Check sheet for the modelled part. Datum: model origin and axes. Units: mm. A direction names the side the tool comes from. Give positions to 0.01 mm unless a question says otherwise; leave off trailing zeros. Write each loop counter-clockwise with the first axis right and the second up, starting at its lowest first coordinate (ties: lowest second). Pieces come first, ordered by that corner, then holes. Notation, with made-up numbers: (-21.75, 29) -> (9.25, 29) arc R23 ccw to (9.25, 54) -> close; hole circle Ø3 at (34, 50). An arc over 180 degrees is marked (long way). Return JSON: item names as keys, results as strings.
from build123d import *

# Parameters (mm, degrees)
BOSS_EXTRUDE1_DEPTH            = 12
SKETCH41_R                     = 1.71
CUT_EXTRUDE7_DEPTH             = 18
CBORE_FOR_M3_SHCS1_D           = 3.4
CBORE_FOR_M3_SHCS1_CBORE_D     = 6.5
CBORE_FOR_M3_SHCS1_CBORE_DEPTH = 3
CBORE_FOR_M3_SHCS2_D           = 3.4
CBORE_FOR_M3_SHCS2_CBORE_D     = 6.5
CBORE_FOR_M3_SHCS2_CBORE_DEPTH = 3
CUT_EXTRUDE10_DEPTH            = 15
CUT_EXTRUDE10_DEPTH_BACK       = 15
SKETCH52_R                     = 1.7
SKETCH58_R                     = 3.25
CUT_EXTRUDE11_DEPTH            = 8
CUT_EXTRUDE12_DEPTH            = 4
CUT_EXTRUDE12_DEPTH_BACK       = 6
FILLET1_R                      = 2
SKETCH61_R                     = 3.25
CUT_EXTRUDE13_DEPTH            = 6
CUT_EXTRUDE14_DEPTH            = 1


with BuildPart() as part:
    # Sketch1 → Boss-Extrude1 (new body)
    with BuildSketch(Plane(origin=(0, 0, 0), x_dir=(0, 1, 0), z_dir=(0, 0, 1))):
        with BuildLine():
            Line((-6.350852961, -13), (13.279056191, -13))
            Line((13.279056191, -13), (13.279056191, -1))
            Line((13.279056191, -1), (3.97617907, -1))
            ThreePointArc((3.97617907, -1), (3.601659304, -1.959094244), (3, -2.794637722))
            Line((3, -2.794637722), (-3, -2.794637722))
            ThreePointArc((-3, -2.794637722), (-3.815101571, -1.501665742), (-4.1, 0))
            ThreePointArc((-4.1, 0), (-0.503818326, 4.06892702), (3.97617907, 1))
            Line((3.97617907, 1), (13.279056191, 1))
            Line((13.279056191, 1), (13.279056191, 13))
            Line((13.279056191, 13), (-6.350852961, 13))
            Line((-6.350852961, 13), (-13.856406461, 0))
            Line((-13.856406461, 0), (-6.350852961, -13))
        make_face()
    extrude(amount=BOSS_EXTRUDE1_DEPTH)

    # Sketch41 → Cut-Extrude7 (cut)
    with BuildSketch(Plane(origin=(0, 0, 0), x_dir=(0, 1, 0), z_dir=(0, 0, 1))):
        with Locations(Location((0, 8.6, 0), (0, 0, 270))):
            Circle(SKETCH41_R)
        with Locations(Location((0, -8.6, 0), (0, 0, 270))):
            Circle(SKETCH41_R)
    extrude(amount=CUT_EXTRUDE7_DEPTH, mode=Mode.SUBTRACT)

    # CBORE for M3 SHCS1 (through all)
    with Locations(Plane(origin=(-8.6, 0, 12), x_dir=(1, 0, 0), z_dir=(0, 0, 1))):
        with Locations((0, 0)):
            CounterBoreHole(CBORE_FOR_M3_SHCS1_D / 2, CBORE_FOR_M3_SHCS1_CBORE_D / 2, CBORE_FOR_M3_SHCS1_CBORE_DEPTH)

    # CBORE for M3 SHCS2 (through all)
    with Locations(Plane(origin=(8.6, 0, 12), x_dir=(1, 0, 0), z_dir=(0, 0, 1))):
        with Locations((0, 0)):
            CounterBoreHole(CBORE_FOR_M3_SHCS2_D / 2, CBORE_FOR_M3_SHCS2_CBORE_D / 2, CBORE_FOR_M3_SHCS2_CBORE_DEPTH)

    # Sketch52 → Cut-Extrude10 (cut, two sides: drawn at the far end of the back side and taken through both)
    with BuildSketch(Plane.YZ.offset(-1).offset(-CUT_EXTRUDE10_DEPTH_BACK)):
        with Locations((8.106406461, 6)):
            Circle(SKETCH52_R)
    extrude(amount=CUT_EXTRUDE10_DEPTH + CUT_EXTRUDE10_DEPTH_BACK, mode=Mode.SUBTRACT)

    # Sketch58 → Cut-Extrude11 (cut)
    with BuildSketch(Plane.YZ.offset(13)):
        with Locations(Location((8.106406461, 6, 0), (0, 0, 270))):
            Circle(SKETCH58_R)
    extrude(amount=-CUT_EXTRUDE11_DEPTH, mode=Mode.SUBTRACT)

    # Sketch60 → Cut-Extrude12 (cut, two sides: drawn at the far end of the back side and taken through both)
    with BuildSketch(Plane.YZ.offset(-8).offset(-CUT_EXTRUDE12_DEPTH_BACK)):
        Polygon((8.106406461, 2.709103466), (10.956406461, 4.354551733), (10.956406461, 7.645448267), (8.106406461, 9.290896534), (5.256406461, 7.645448267), (5.256406461, 4.354551733), align=None)
    extrude(amount=CUT_EXTRUDE12_DEPTH + CUT_EXTRUDE12_DEPTH_BACK, mode=Mode.SUBTRACT)

    # Fillet1
    # the kernel refuses this fillet: 2 mm, written as the material it takes off along each edge
    with BuildSketch(Plane(origin=(13, 13.279056191, -5), x_dir=(0, -1, 0), z_dir=(0, 0, 1))) as fillet1_piece_1:
        with BuildLine():
            CenterArc((FILLET1_R, -FILLET1_R), FILLET1_R, 90, 90)
            Line((0, -FILLET1_R), (0, 0))
            Line((0, 0), (FILLET1_R, 0))
        make_face()
    extrude(amount=22, mode=Mode.SUBTRACT)
    with BuildSketch(Plane(origin=(-13, 13.279056191, -5), x_dir=(0, -1, 0), z_dir=(0, 0, 1))) as fillet1_piece_2:
        with BuildLine():
            CenterArc((FILLET1_R, FILLET1_R), FILLET1_R, 180, 90)
            Line((0, FILLET1_R), (0, 0))
            Line((0, 0), (FILLET1_R, 0))
        make_face()
    extrude(amount=22, mode=Mode.SUBTRACT)

    # Sketch61 → Cut-Extrude13 (cut)
    with BuildSketch(Plane(origin=(0, 0, 12), x_dir=(0, 1, 0), z_dir=(0, 0, 1))):
        with Locations(Location((0, 8.6, 0), (0, 0, 270))):
            Circle(SKETCH61_R)
        with Locations(Location((0, -8.6, 0), (0, 0, 270))):
            Circle(SKETCH61_R)
    extrude(amount=-CUT_EXTRUDE13_DEPTH, mode=Mode.SUBTRACT)

    # Sketch62 → Cut-Extrude14 (cut)
    with BuildSketch(Plane(origin=(-6, -10.392304845, 0), x_dir=(0.8660254037844386, -0.5000000000000001, 0), z_dir=(-0.5000000000000001, -0.8660254037844386, 0))):
        with BuildLine():
            Line((1.681473513, 6.646959362), (1.681473513, 6.287985003))
            Line((1.681473513, 6.287985003), (0.491669827, 6.287985003))
            Line((0.491669827, 6.287985003), (0.302366943, 5.367412086))
            add(Edge.make_bspline(
                [(0.302366943, 5.367412086), (0.339422817, 5.377642358), (0.411212713, 5.397461892), (0.517172574, 5.419467662), (0.617764777, 5.432733106), (0.683040148, 5.434544417), (0.714626558, 5.435420901)],
                knots=[0, 0, 0, 0, 1.100273476, 2.13160584, 3.095893838, 4, 4, 4, 4], degree=3))
            add(Edge.make_bspline(
                [(0.714626558, 5.435420901), (0.753710298, 5.434574965), (0.830558695, 5.432911644), (0.942997642, 5.416939795), (1.050330535, 5.39179988), (1.152332906, 5.356679358), (1.249193456, 5.311769625), (1.340021018, 5.255669685), (1.426178931, 5.190136353), (1.506121525, 5.114791341), (1.578645833, 5.031869725), (1.642411822, 4.942711854), (1.696574413, 4.848184192), (1.740135168, 4.747383583), (1.774919502, 4.641424429), (1.798071497, 4.529191847), (1.813488206, 4.411743727), (1.815210592, 4.331439157), (1.816088898, 4.29048901)],
                knots=[0, 0, 0, 0, 1.052922333, 2.070308379, 3.05430497, 4.020497103, 4.973039431, 5.925935799, 6.892292201, 7.88610001, 8.88166317, 9.857072816, 10.836096531, 11.812156883, 12.81219415, 13.836441305, 14.89672472, 16, 16, 16, 16], degree=3))
            add(Edge.make_bspline(
                [(1.816088898, 4.29048901), (1.815423823, 4.261966789), (1.81410266, 4.205307802), (1.807384072, 4.121163601), (1.794448356, 4.038800768), (1.777080632, 3.958208376), (1.754538214, 3.879539004), (1.72724916, 3.802567476), (1.693853133, 3.727772869), (1.657221758, 3.654447474), (1.61597528, 3.584248967), (1.570196772, 3.51859998), (1.521831281, 3.456515699), (1.469789896, 3.398661966), (1.4135889, 3.345418948), (1.353908934, 3.296470667), (1.291226215, 3.250989336), (1.224570972, 3.210821141), (1.155428489, 3.173858185), (1.082800272, 3.143534648), (1.008339572, 3.116424119), (0.930974696, 3.094814592), (0.850880883, 3.077882037), (0.767926108, 3.066381437), (0.682545438, 3.058004999), (0.624670425, 3.057480642), (0.595435853, 3.057215772)],
                knots=[0, 0, 0, 0, 1.056347294, 2.098418968, 3.122841568, 4.141288669, 5.149314143, 6.15115421, 7.162517403, 8.180376062, 9.185164535, 10.17417709, 11.141909838, 12.097768115, 13.052685741, 14.0056014, 14.954263652, 15.917497458, 16.885230207, 17.854509472, 18.828990115, 19.81800267, 20.826176721, 21.857883937, 22.917946725, 24, 24, 24, 24], degree=3))
            add(Edge.make_bspline(
                [(0.595435853, 3.057215772), (0.560561672, 3.05790661), (0.491950842, 3.059265752), (0.391430275, 3.073484238), (0.294715669, 3.093848154), (0.202585568, 3.124484424), (0.114214304, 3.162871719), (0.030791586, 3.21138789), (-0.04981419, 3.266366994), (-0.124326227, 3.331247347), (-0.19348234, 3.402163029), (-0.255388849, 3.47912067), (-0.310522426, 3.560850112), (-0.358000173, 3.647748266), (-0.398498194, 3.739586797), (-0.430313182, 3.836709798), (-0.455991537, 3.938609802), (-0.466854958, 4.008763312), (-0.472372641, 4.04439526)],
                knots=[0, 0, 0, 0, 1.0467383, 2.05933395, 3.04377827, 4.011590433, 4.970194871, 5.932262533, 6.905835911, 7.896367577, 8.894135286, 9.877477877, 10.858688626, 11.851381753, 12.8477658, 13.868841284, 14.917554742, 16, 16, 16, 16], degree=3))
            Line((-0.472372641, 4.04439526), (-0.158270076, 4.04439526))
            add(Edge.make_bspline(
                [(-0.158270076, 4.04439526), (-0.150541519, 4.011018807), (-0.135686803, 3.946867412), (-0.103081054, 3.856736071), (-0.063215178, 3.776416847), (-0.01581083, 3.704847264), (0.040739201, 3.642438267), (0.105268629, 3.586821205), (0.177616353, 3.536646075), (0.258009582, 3.494823308), (0.342822662, 3.459154555), (0.431589872, 3.43540286), (0.521894218, 3.418701967), (0.582972588, 3.417030206), (0.61366502, 3.416190131)],
                knots=[0, 0, 0, 0, 1.136247022, 2.183929868, 3.172523383, 4.106158343, 5.02341133, 5.958108904, 6.928429099, 7.938127109, 8.96079061, 9.975095812, 10.982467395, 12, 12, 12, 12], degree=3))
            add(Edge.make_bspline(
                [(0.61366502, 3.416190131), (0.643623464, 3.417010909), (0.702611886, 3.418627028), (0.789423273, 3.43106604), (0.873236147, 3.450223611), (0.953223504, 3.478893466), (1.030785044, 3.513738184), (1.103958814, 3.55845326), (1.174861691, 3.609913279), (1.241289825, 3.668869909), (1.302129274, 3.733839603), (1.355885395, 3.803316997), (1.400662308, 3.877433843), (1.438396417, 3.954906996), (1.467049716, 4.036585553), (1.487490697, 4.122086729), (1.499493756, 4.211621709), (1.501144936, 4.272691019), (1.501986334, 4.303810324)],
                knots=[0, 0, 0, 0, 1.027316725, 2.022795036, 3.002884548, 3.971462791, 4.93288096, 5.914575861, 6.907176829, 7.935150275, 8.956128384, 9.956726525, 10.942570165, 11.921478529, 12.907843606, 13.90538589, 14.932640048, 16, 16, 16, 16], degree=3))
            add(Edge.make_bspline(
                [(1.501986334, 4.303810324), (1.501327854, 4.331886075), (1.500038975, 4.386840364), (1.489508404, 4.467239571), (1.471191432, 4.543312613), (1.445767552, 4.615426847), (1.413488044, 4.683650289), (1.374041732, 4.74805335), (1.326688334, 4.807787183), (1.272596445, 4.862879736), (1.213338404, 4.913724611), (1.147894662, 4.957068698), (1.077634735, 4.993532615), (1.003405136, 5.025000614), (0.923440237, 5.047601359), (0.839323605, 5.064569245), (0.750146897, 5.074384607), (0.689176208, 5.075746496), (0.657835693, 5.076446542)],
                knots=[0, 0, 0, 0, 1.045622112, 2.046656509, 3.013763289, 3.955457236, 4.890082067, 5.820317437, 6.762574623, 7.722996705, 8.69280354, 9.665887285, 10.63943826, 11.638615906, 12.663482002, 13.728887084, 14.832589034, 16, 16, 16, 16], degree=3))
            add(Edge.make_bspline(
                [(0.657835693, 5.076446542), (0.630706764, 5.07586595), (0.574692409, 5.074667177), (0.488769582, 5.06584068), (0.398477859, 5.051601386), (0.304163363, 5.032015138), (0.205542855, 5.006384062), (0.102824455, 4.975669561), (-0.004207812, 4.938947562), (-0.076325536, 4.911215348), (-0.113398282, 4.896959362)],
                knots=[0, 0, 0, 0, 0.817624296, 1.688186739, 2.600797293, 3.572016777, 4.590301741, 5.671205678, 6.80286297, 8, 8, 8, 8], degree=3))
            Line((-0.113398282, 4.896959362), (0.245576077, 6.646959362))
            Line((0.245576077, 6.646959362), (1.681473513, 6.646959362))
        make_face()
    extrude(amount=-CUT_EXTRUDE14_DEPTH, mode=Mode.SUBTRACT)


solid = part.part
(1) Cross-section at C-C on x = 8.6. Enter the section's corners in (y, z), then the cut area to 3 significant figures.
Reply:
{"outline": "(-8.89, 0) -> (-1.71, 0) -> (-1.71, 6) -> (-3.25, 6) -> (-3.25, 12) -> (-8.89, 12) -> close; (1.71, 0) -> (13.28, 0) -> (13.28, 12) -> (3.25, 12) -> (3.25, 6) -> (1.71, 6) -> close; hole circle Ø6.5 at (8.11, 6)", "area": "173 mm^2"}
(2) Thickness scan on L1, parallel to X at y = 4.75, z = 2.25; L2, parallel to Y at x = -9, z = 8; L3, parallel to X at y = 11, z = 6. Record the ranges inside material, lowest first.
Reply:
{"L1": "-13 to -1, 1 to 13", "L2": "-8.66 to -3.23, 3.23 to 5.87, 10.34 to 13.28", "L3": "-13 to -1, 1 to 5"}
(3) Release check for a two-part mould opening along Y. For faces 1 (the flat face through (5, 6.7, 4.6)), 2 (the flat face through (-6.59, -10.05, 5.92)), 3 (the flat face through (2.795, 0, 6)), 4 (the flat face through (-13, 3, 6)) record: pulls with the +Y half, pulls with the -Y half, needs draft (parallel to the pull), parting line crosses it, or undercut.
Reply:
{"face 1": "undercut", "face 2": "pulls with the -Y half", "face 3": "undercut", "face 4": "needs draft"}
(4) Depth check by flat-ended pin: pin 1 Ø2 at (y, z) = (8.11, 6) entering from -X; pin 2 Ø5 at (x, z) = (-1.5, 7.5) entering from -Y; pin 3 Ø3 at (y, z) = (8.5, 5.5) entering from -X; pin 4 Ø2.5 at (x, z) = (-8, 6) entering from -Y. Enter the tip coordinate at first touch or a pass-through.
Reply:
{"pin 1": "through", "pin 2": "y = -13.86", "pin 3": "x = -4", "pin 4": "y = -9.96"}
(5) Cross-section at D-D on z = 9.75. Enter the section's corners in (x, y), then the cut area to 3 significant figures.
Reply:
{"outline": "(-13, -6.35) -> (0, -13.86) -> (13, -6.35) -> (13, 11.28) arc R2 ccw to (11, 13.28) -> (1, 13.28) -> (1, 3.98) arc R4.1 cw to (2.79, 3) -> (2.79, -3) arc R4.1 cw (long way) to (-1, 3.98) -> (-1, 13.28) -> (-11, 13.28) arc R2 ccw to (-13, 11.28) -> close; hole circle Ø6.5 at (-8.6, 0); hole circle Ø6.5 at (8.6, 0)", "area": "474 mm^2"}
(6) Cross-section at B-B on x = -7.5. Enter the section's corners in (y, z), then the cut area to 3 significant figures.
Reply:
{"outline": "(-9.53, 0) -> (-1.31, 0) -> (-1.31, 6) -> (-3.06, 6) -> (-3.06, 12) -> (-9.53, 12) -> close; (1.31, 0) -> (13.28, 0) -> (13.28, 12) -> (3.06, 12) -> (3.06, 6) -> (1.31, 6) -> close; hole (5.26, 4.35) -> (8.11, 2.71) -> (10.96, 4.35) -> (10.96, 7.65) -> (8.11, 9.29) -> (5.26, 7.65) -> close", "area": "193 mm^2"}
(7) Set-up check for faces 5 (the flat face through (1, 10, 5)), 6 (the flat face through (-4.8, -10.5, 6.288)), 7 (the flat face through (-8.56, 6.7, 8.48)): record each of +Z, -Z, +X, -X, +Y, -Y from which the full face is reachable in a straight line by a thin tool's end or side.
Reply:
{"face 5": "+Z, -Z, +Y", "face 6": "none", "face 7": "-X"}
(8) Cross-section at A-A on z = 2. Enter the section's corners in (x, y).
Reply:
{"outline": "(-13, -6.35) -> (0, -13.86) -> (13, -6.35) -> (13, 11.28) arc R2 ccw to (11, 13.28) -> (1, 13.28) -> (1, 3.98) arc R4.1 cw to (2.79, 3) -> (2.79, -3) arc R4.1 cw (long way) to (-1, 3.98) -> (-1, 13.28) -> (-11, 13.28) arc R2 ccw to (-13, 11.28) -> close; hole circle Ø3.42 at (-8.6, 0); hole circle Ø3.42 at (8.6, 0)"}
